from build123d import *

# Parameters (mm, degrees)
EXTRUDE_1_DEPTH     = 57.2
SKETCH_2_W          = 2
SKETCH_2_H          = 1.6
EXTRUDE_2_DEPTH     = 57.2
CHAMFER_1_SIZE      = 0.5
SKETCH_3_W          = 46.4
SKETCH_3_H          = 8.2
EXTRUDE_3_DEPTH     = 2
SKETCH_4_W          = 20
SKETCH_4_H          = 10
CUT_EXTRUDE_1_DEPTH = 2
FILLET_1_R          = 1
FILLET_2_R          = 2
SKETCH_5_W          = 2
SKETCH_5_H          = 3
CUT_EXTRUDE_2_DEPTH = 2
EXTRUDE_4_DEPTH     = 1


with BuildPart() as part:
    # 草图1 → 凸台-拉伸1 (new body)
    with BuildSketch(Plane(origin=(0, 0, 0), x_dir=(0, 0, -1), z_dir=(1, 0, 0))):
        Polygon((-3.2, 0), (-0.2, 0), (-0.2, 6.2), (40.2, 6.2), (40.2, 0), (43.2, 0), (43.2, 8.2), (-3.2, 8.2), align=None)
    extrude(amount=EXTRUDE_1_DEPTH)

    # 草图2 → 凸台-拉伸2 (add)
    with BuildSketch(Plane.ZY):
        with Locations((-39.2, 3)):
            Rectangle(SKETCH_2_W, SKETCH_2_H)
        with Locations((-0.8, 3)):
            Rectangle(SKETCH_2_W, SKETCH_2_H)
    extrude(amount=-EXTRUDE_2_DEPTH)

    # 倒角1
    chamfer_1_edges = [part.edges().sort_by_distance(p)[0] for p in [
        (0, 2.2, -39.2),
        (0, 3, -38.2),
        (0, 3.8, -39.2),
        (0, 3.8, -0.8),
        (0, 3, -1.8),
        (0, 2.2, -0.8),
    ]]
    chamfer(chamfer_1_edges, length=CHAMFER_1_SIZE)

    # 草图3 → 凸台-拉伸3 (add)
    with BuildSketch(Plane(origin=(57.2, 0, 0), x_dir=(0, 0, -1), z_dir=(1, 0, 0))):
        with Locations((20, 4.1)):
            Rectangle(SKETCH_3_W, SKETCH_3_H)
    extrude(amount=EXTRUDE_3_DEPTH)

    # 草图4 → 切除-拉伸1 (cut)
    with BuildSketch(Plane(origin=(0, 8.2, 0), x_dir=(1, 0, 0), z_dir=(0, 1, 0))):
        with Locations((14, 9.8)):
            Rectangle(SKETCH_4_W, SKETCH_4_H)
    extrude(amount=-CUT_EXTRUDE_1_DEPTH, mode=Mode.SUBTRACT)

    # 圆角1
    fillet_1_edges = [part.edges().sort_by_distance(p)[0] for p in [
        (29.6, 8.2, 3.2),
        (29.6, 8.2, -43.2),
        (0, 4.1, 3.2),
        (0, 8.2, -20),
        (0, 4.1, -43.2),
        (59.2, 4.1, 3.2),
        (59.2, 4.1, -43.2),
        (59.2, 8.2, -20),
    ]]
    fillet(fillet_1_edges, radius=FILLET_1_R)

    # 圆角2
    fillet_2_edges = [part.edges().sort_by_distance(p)[0] for p in [
        (4, 7.2, -4.8),
        (4, 7.2, -14.8),
        (24, 7.2, -14.8),
        (24, 7.2, -4.8),
    ]]
    fillet(fillet_2_edges, radius=FILLET_2_R)

    # 草图5 → 切除-拉伸2 (cut)
    with BuildSketch(Plane(origin=(0, 8.2, 0), x_dir=(1, 0, 0), z_dir=(0, 1, 0))):
        with Locations((2.5, 20)):
            Rectangle(SKETCH_5_W, SKETCH_5_H)
    extrude(amount=-CUT_EXTRUDE_2_DEPTH, mode=Mode.SUBTRACT)

    # 草图6 → 凸台-拉伸4 (add)
    # profile 1 of 3: a face of its own
    with BuildSketch(Plane(origin=(0, 8.2, 0), x_dir=(1, 0, 0), z_dir=(0, 1, 0))):
        with BuildLine():
            Line((43.210238434, 27.609218662), (46.004565148, 29.278219616))
            Line((46.004565148, 29.278219616), (41.153736267, 31.052319712))
            add(Edge.make_bspline(
                [(41.153736267, 31.052319712), (38.917601784, 31.936798518), (38.081456616, 32.783594578), (37.429599552, 34.039752086), (37.178253479, 34.799893267)],
                knots=[0, 0, 0, 0, 0.258597765, 0.606503624, 0.606503624, 0.606503624, 0.606503624], degree=3))
            add(Edge.make_bspline(
                [(37.178253479, 34.799893267), (27.495556624, 37.127469308), (28.540823689, 37.034185208), (22.273471515, 38.064657168), (21.101157932, 38.034742746)],
                knots=[0, 0, 0, 0, 0.625762474, 1, 1, 1, 1], degree=3))
            add(Edge.make_bspline(
                [(21.101157932, 38.034742746), (26.275616415, 37.491858388), (30.685853804, 34.799893267)],
                knots=[0, 0, 0, 1, 1, 1], degree=2))
            add(Edge.make_bspline(
                [(30.685853804, 34.799893267), (32.176490653, 33.72226655), (30.681444749, 32.541026773)],
                knots=[0, 0, 0, 1, 1, 1], degree=2))
            Line((30.681444749, 32.541026773), (13.273453583, 19.243046464))
            add(Edge.make_bspline(
                [(13.273453583, 19.243046464), (27.82860145, 28.923958356), (43.210238434, 27.609218662)],
                knots=[0, 0, 0, 0.904008086, 0.904008086, 0.904008086], degree=2))
        make_face()
        Polygon((36.709764713, 30.912438237), (37.178253479, 29.699300691), (39.856659814, 29.454156879), align=None, mode=Mode.SUBTRACT)
    # profile 2 of 3: a face of its own
    with BuildSketch(Plane(origin=(0, 8.2, 0), x_dir=(1, 0, 0), z_dir=(0, 1, 0))):
        with BuildLine():
            Line((29.392459455, 32.336818489), (27.193702695, 30.773846816))
            add(Edge.make_bspline(
                [(19.299371197, 32.177872217), (23.346710302, 32.024077211), (27.193702695, 30.773846816)],
                knots=[0, 0, 0, 1, 1, 1], degree=2))
            add(Edge.make_bspline(
                [(19.299371197, 32.177872217), (24.339492566, 32.815798813), (29.392459455, 32.336818489)],
                knots=[0, 0, 0, 1, 1, 1], degree=2))
        make_face()
    # profile 3 of 3: a face of its own
    with BuildSketch(Plane(origin=(0, 8.2, 0), x_dir=(1, 0, 0), z_dir=(0, 1, 0))):
        Polygon((16.46482935, 26.694225841), (24.730035483, 28.8929826), (22.359389371, 27.082043876), align=None)
    extrude(amount=EXTRUDE_4_DEPTH)


solid = part.part
Input: part model. Units: mm. Frame: model coordinates. A direction names the side the tool comes from. Coordinates: 2 decimals unless noted, no trailing zeros. Loops run counter-clockwise (first coordinate to the right, second up) from the corner with the lowest first, then second, coordinate; pieces in that order, holes last. Notation, with made-up numbers: (39.5, 65.5) - (90.5, 65.5) arc R18 cw to (90.5, 76.5) - close; hole circle Ø1 at (49.5, -27.75). An arc over 180 degrees is marked (long way). Answer in a Markdown table with one row per item. Add a question column.
Item 1: Section query B-B on x = 9. Return the cut outline in (y, z), then the cut area to 3 significant figures.
Item 2: Access query for faces 1 (the flat face through (20.54, 8.69, -27.78)), 2 (the flat face through (23.56, 8.69, -28)), 3 (the flat face through (28, 2.2, -39)), 4 (the flat face through (28, 5, -40.2)). Directions: +Z, -Z, +X, -X, +Y, -Y. A direction counts if a zero-diameter tool reaches every point of the face in a straight line with its end or side. Return the directions, or none.
Item 3: Section query C-C on y = 5.25. Return the cut outline in (x, z).
Item 4: Section query D-D on z = -4. Return the cut outline in (x, y).
Item 5: Line query: line 1 along Z through (x, y) = (54, 4.25); line 2 along Z through (x, y) = (8, 6.5); line 3 along Y through (x, z) = (16, -0.5). Output: solid intervals per line, ascending. Write a range as [from, to].
Item 6: Section query A-A on z = -12. Return the cut outline in (x, y), then the cut area to 3 significant figures.
Item 7: Contact query for flat-ended pins moving along their axis: P1, Ø0.6, axis at y = 7.5, z = -9, coming from the -X side; P2, Ø1, axis at x = 16, z = -1, coming from the -Y side; P3, Ø6, axis at x = 25.5, z = -5.5, coming from the +Y side; P4, Ø10, axis at x = 51.5, z = -20, coming from the -Y side. Output: stop coordinate, or through.
Item 8: Mould query, pull axis Z, two halves, no side actions, for faces 5 (the flat face through (0, 7, -20)), 6 (the flat face through (43.613, 8.693, -30.153)), 7 (the cylindrical face through (23.4, 7.19, -5.37)). Classes: released by +Z, released by -Z, zero draft, split by the parting line, or undercut.
Recorded:
| question | item | result |
|---|---|---|
| 1 | outline | (0, -43.2) - (7.2, -43.2) arc R1 ccw to (8.2, -42.2) - (8.2, -14.8) - (6.2, -14.8) - (6.2, -40.2) - (3.8, -40.2) - (3.8, -38.2) - (2.2, -38.2) - (2.2, -40.2) - (0, -40.2) - close; (0, 0.2) - (2.2, 0.2) - (2.2, -1.8) - (3.8, -1.8) - (3.8, 0.2) - (6.2, 0.2) - (6.2, -4.8) - (8.2, -4.8) - (8.2, 2.2) arc R1 ccw to (7.2, 3.2) - (0, 3.2) - close |
| 1 | area | 116 mm^2 |
| 2 | face 1 | -X, +Y |
| 2 | face 2 | +Y |
| 2 | face 3 | -X, -Y |
| 2 | face 4 | -X |
| 3 | outline | (0, -42.2) arc R1 ccw to (1, -43.2) - (58.2, -43.2) arc R1 ccw to (59.2, -42.2) - (59.2, 2.2) arc R1 ccw to (58.2, 3.2) - (1, 3.2) arc R1 ccw to (0, 2.2) - (0, 0.2) - (57.2, 0.2) - (57.2, -40.2) - (0, -40.2) - close |
| 4 | outline | (0, 6.2) - (57.2, 6.2) - (57.2, 0) - (59.2, 0) - (59.2, 7.2) arc R1 ccw to (58.2, 8.2) - (1, 8.2) arc R1 ccw to (0, 7.2) - close |
| 5 | line 1 | [-43.2, -40.2], [0.2, 3.2] |
| 5 | line 2 | [-43.2, -14.8], [-4.8, 3.2] |
| 5 | line 3 | [2.2, 3.8], [6.2, 8.2] |
| 6 | outline | (0, 6.2) - (4, 6.2) - (4, 8.2) - (1, 8.2) arc R1 ccw to (0, 7.2) - close; (24, 6.2) - (57.2, 6.2) - (57.2, 0) - (59.2, 0) - (59.2, 7.2) arc R1 ccw to (58.2, 8.2) - (24, 8.2) - close |
| 6 | area | 90.4 mm^2 |
| 7 | P1 | x = 0 |
| 7 | P2 | y = 2.2 |
| 7 | P3 | y = 8.2 |
| 7 | P4 | y = 6.2 |
| 8 | face 5 | zero draft |
| 8 | face 6 | released by -Z |
| 8 | face 7 | undercut |
